Verification items for the finished model (mm, model axes). A direction names the side the tool comes from. Coordinates: 2 decimals unless noted, no trailing zeros. Write each loop counter-clockwise with the first axis right and the second up, starting at its lowest first coordinate (ties: lowest second). Pieces come first, ordered by that corner, then holes. Notation, with made-up numbers: (7, 39.5) -> (51, 39.5) arc R3 ccw to (51, 43.5) -> close; hole circle Ø11 at (29, 35.5). An arc over 180 degrees is marked (long way). Use CSV: the item, a comma, the result in double quotes.
```python
from build123d import *

# Parameters (mm, degrees)
BOSS_EXTRUDE2_REACH                                  = 123.758
SKETCH4_119_W                                        = 22
SKETCH4_119_H                                        = 60
BOSS_EXTRUDE3_DEPTH                                  = 50
CUT_EXTRUDE1_DEPTH                                   = 20
CUT_EXTRUDE2_DEPTH                                   = 50
CUT_EXTRUDE3_START                                   = -10
SKETCH4_121_W                                        = 20
SKETCH4_121_H                                        = 60
SKETCH4_121_W_2                                      = 22
CUT_EXTRUDE3_DEPTH                                   = 10
CBORE_FOR_5_16_BINDING_HEAD_MACHINE_SCRE_D           = 5.499999922
CBORE_FOR_5_16_BINDING_HEAD_MACHINE_SCRE_DEPTH       = 30
CBORE_FOR_5_16_BINDING_HEAD_MACHINE_SCRE_CBORE_D     = 12.239999904
CBORE_FOR_5_16_BINDING_HEAD_MACHINE_SCRE_CBORE_DEPTH = 3.579999952
CBORE_FOR_5_16_BINDING_HEAD_MACHINE_SCRE_TIP         = 1.652366679


with BuildPart() as part:
    # Loft3: read off the stored shape, not the designer's step
    # Loft3: loft between two sections, ruled curve by curve
    loft3_from = [
        Edge.make_bspline([(-25, 20, 30), (0, 20, 0)], [0, 0, 1, 1], 1),
        Edge.make_bspline([(0, 20, 0), (-25, 20, -30)], [0, 0, 1, 1], 1),
        Edge.make_line((-73, 20, 30), (-25, 20, 30)),
        Edge.make_line((-25, 20, -30), (-73, 20, -30)),
        Edge.make_line((-73, 20, -30), (-73, 20, 30)),
    ]
    loft3_to = [
        Edge.make_bspline([(-73, 70, 30), (-64, 70, 0)], [0, 0, 1, 1], 1),
        Edge.make_bspline([(-64, 70, 0), (-73, 70, -30)], [0, 0, 1, 1], 1),
        Edge.make_line((-95, 70, 30), (-73, 70, 30)),
        Edge.make_line((-73, 70, -30), (-95, 70, -30)),
        Edge.make_line((-95, 70, -30), (-95, 70, 30)),
    ]
    loft3 = Solid(Shell([*[Face.make_surface_from_curves(loft3_from[k], loft3_to[k]) for k in range(5)], Face(Wire(loft3_from)), Face(Wire(loft3_to))]))
    add(loft3)

    # Boss-Extrude2: up to this face of the body (flat: up to its plane)
    boss_extrude2_end = Plane(part.part.faces().sort_by_distance((-42.319559229, 20, 0))[0])
    # Sketch1 → Boss-Extrude2 (add, up to the picked face)
    with BuildSketch(Plane(origin=(0, 0, 0), x_dir=(1, 0, 0), z_dir=(0, 1, 0)), mode=Mode.PRIVATE) as boss_extrude2_sk1:
        Polygon((-115, -30), (-115, 30), (-25, 30), (0, 0), (-25, -30), align=None)
    boss_extrude2_tool1 = split(extrude(boss_extrude2_sk1.sketch, amount=BOSS_EXTRUDE2_REACH, mode=Mode.PRIVATE), bisect_by=boss_extrude2_end, keep=Keep.BOTH, mode=Mode.PRIVATE)
    add(boss_extrude2_tool1.solids().sort_by(Axis((-63.495935, 0, 0), (0, 1, 0)))[0])

    # Sketch4 → Loft7 section 0
    with BuildSketch(Plane(origin=(0, 20, 0), x_dir=(1, 0, 0), z_dir=(0, 1, 0))):
        with BuildLine():
            Line((-73, -30), (-73, 30))
            Line((-73, 30), (-95, 30))
            Line((-95, 30), (-95, -30))
            Line((-95, -30), (-73, -30))
        make_face()
    # Sketch2<11> → Loft7 section 1
    with BuildSketch(Plane(origin=(0, 70, 0), x_dir=(1, 0, 0), z_dir=(0, 1, 0))):
        with BuildLine():
            Line((-115, 10), (-115, -10))
            Line((-115, -10), (-95, -10))
            Line((-95, -10), (-95, 10))
            Line((-95, 10), (-115, 10))
        make_face()
    loft()

    # Sketch2<14> → section 1 of loft9
    with BuildSketch(Plane(origin=(0, 70, 0), x_dir=(1, 0, 0), z_dir=(0, 1, 0)), mode=Mode.PRIVATE) as loft9_s1:
        with BuildLine():
            Line((-115, 10), (-115, -10))
            Line((-115, -10), (-95, -10))
            Line((-95, -10), (-95, 10))
            Line((-95, 10), (-115, 10))
        make_face()
    # loft from a face of the part (loft9)
    loft([part.faces().sort_by_distance((-105, 20, 0))[0], loft9_s1.sketch])

    # Sketch4<119> → Boss-Extrude3 (add)
    with BuildSketch(Plane(origin=(0, 20, 0), x_dir=(1, 0, 0), z_dir=(0, 1, 0))):
        with Locations((-84, 0)):
            Rectangle(SKETCH4_119_W, SKETCH4_119_H)
    extrude(amount=BOSS_EXTRUDE3_DEPTH)

    # Sketch2<8> → Cut-Extrude1 (cut)
    with BuildSketch(Plane(origin=(0, 70, 0), x_dir=(1, 0, 0), z_dir=(0, 1, 0))):
        with BuildLine():
            Line((-89, 19.903363007), (-89, -16.052534228))
            ThreePointArc((-89, -16.052534228), (-81, -24.052534228), (-73, -16.052534228))
            Line((-73, -16.052534228), (-73, 19.903363007))
            ThreePointArc((-73, 19.903363007), (-81, 27.903363007), (-89, 19.903363007))
        make_face()
        with BuildLine():
            ThreePointArc((-78, 19.903363007), (-81, 22.903363007), (-84, 19.903363007))
            Line((-84, 19.903363007), (-84, -16.052534228))
            ThreePointArc((-84, -16.052534228), (-81, -19.052534228), (-78, -16.052534228))
            Line((-78, -16.052534228), (-78, 19.903363007))
        make_face(mode=Mode.SUBTRACT)
    extrude(amount=-CUT_EXTRUDE1_DEPTH, mode=Mode.SUBTRACT)

    # Sketch2<13> → Cut-Extrude2 (cut)
    with BuildSketch(Plane(origin=(0, 70, 0), x_dir=(1, 0, 0), z_dir=(0, 1, 0))):
        with BuildLine():
            Line((-78, -16.052534228), (-78, 19.903363007))
            ThreePointArc((-78, 19.903363007), (-81, 22.903363007), (-84, 19.903363007))
            Line((-84, 19.903363007), (-84, -16.052534228))
            ThreePointArc((-84, -16.052534228), (-81, -19.052534228), (-78, -16.052534228))
        make_face()
    extrude(amount=-CUT_EXTRUDE2_DEPTH, mode=Mode.SUBTRACT)

    # Sketch4<121> → Cut-Extrude3 (cut)
    with BuildSketch(Plane(origin=(0, 20, 0), x_dir=(1, 0, 0), z_dir=(0, 1, 0)).offset(CUT_EXTRUDE3_START)):
        with Locations((-105, 0)):
            Rectangle(SKETCH4_121_W, SKETCH4_121_H)
        with Locations((-84, 0)):
            Rectangle(SKETCH4_121_W_2, SKETCH4_121_H)
    extrude(amount=-CUT_EXTRUDE3_DEPTH, mode=Mode.SUBTRACT)

    # CBORE for 5/16 Binding Head Machine Screw1
    with Locations(Plane(origin=(0, 70, 0), x_dir=(1, 0, 0), z_dir=(0, 1, 0))):
        with Locations((-105.496950166, 0)):
            CounterBoreHole(CBORE_FOR_5_16_BINDING_HEAD_MACHINE_SCRE_D / 2, CBORE_FOR_5_16_BINDING_HEAD_MACHINE_SCRE_CBORE_D / 2, CBORE_FOR_5_16_BINDING_HEAD_MACHINE_SCRE_CBORE_DEPTH, depth=CBORE_FOR_5_16_BINDING_HEAD_MACHINE_SCRE_DEPTH)
            with Locations((0, 0, -(CBORE_FOR_5_16_BINDING_HEAD_MACHINE_SCRE_DEPTH + CBORE_FOR_5_16_BINDING_HEAD_MACHINE_SCRE_TIP / 2))):  # 118° drill point
                Cone(0, CBORE_FOR_5_16_BINDING_HEAD_MACHINE_SCRE_D / 2, CBORE_FOR_5_16_BINDING_HEAD_MACHINE_SCRE_TIP, mode=Mode.SUBTRACT)


solid = part.part
```
1) Gauge pin test, flat ends, axial feed: pin 1 (21 mm diameter, centred on x = -99, z = 10.5, fed in from -Y); pin 2 (9 mm diameter, centred on y = 34.5, z = -1.5, fed in from +X); pin 3 (3 mm diameter, centred on x = -81.5, z = 5, fed in from +Y). Record the tip position at first contact, or that the pin passes through.
Return value:
pin 1,"y = 10"
pin 2,"x = -13.13"
pin 3,"y = 20"
2) Mould release check, pull along Z, two halves, no side actions. Record for faces 1 (the flat face through (-77.6, 50, -2.3)), 2 (the flat face through (-95, 56, -24)), 3 (the flat face through (-84, 35, -2)), 4 (the flat face through (-71, 27, -30)): released by +Z, released by -Z, zero draft, split by the parting line, or undercut.
Return value:
face 1,"undercut"
face 2,"zero draft"
face 3,"undercut"
face 4,"released by -Z"
3) Cross-section at B-B (y = 52.5). Give the number of separate pieces and of enclosed holes in the cut face, plus the area to 3 significant figures.
Return value:
separate pieces,"1"
enclosed holes,"2"
area,"2,650 mm2"
4) Cross-section at A-A (x = -81). Record the boundary of the cut face in (y, z), plus the area to 3 significant figures.
Return value:
outline,"(10, -30) -> (70, -30) -> (70, -27.9) -> (50, -27.9) -> (50, -22.9) -> (20, -22.9) -> (20, 19.05) -> (50, 19.05) -> (50, 24.05) -> (70, 24.05) -> (70, 30) -> (10, 30) -> close"
area,"1,300 mm2"
5) Cross-section at C-C (y = 15). Record the boundary of the cut face in (x, z).
Return value:
outline,"(-115, -30) -> (-25, -30) -> (0, 0) -> (-25, 30) -> (-115, 30) -> close"
6) Scan lines: L1, parallel to X at y = 56, z = 7; L2, parallel to Y at x = -87, z = -1.5; L3, parallel to Z at x = -78.5, y = 28. Record each from-to range of solid material in increasing order.
Return value:
L1,"-115 to -89, -73 to -49.23"
L2,"10 to 50"
L3,"-30 to -21.56, 17.71 to 30"
7) Set-up check for faces 5 (the flat face through (-115, 34, 0)), 6 (the flat face through (-91, 70, 2)), 7 (the flat face through (-105, 45, 20)), 8 (the flat face through (-73, 5, 0)), 9 (the cylindrical face through (-81.07, 35.21, 19.05)): record each of +Z, -Z, +X, -X, +Y, -Y from which the full face is reachable in a straight line by a thin tool's end or side.
Return value:
face 5,"+Z, -Z, -X, +Y, -Y"
face 6,"+Z, -Z, +X, -X, +Y"
face 7,"+Z, -X, +Y"
face 8,"+Z, -Z, -X, -Y"
face 9,"+Y"
